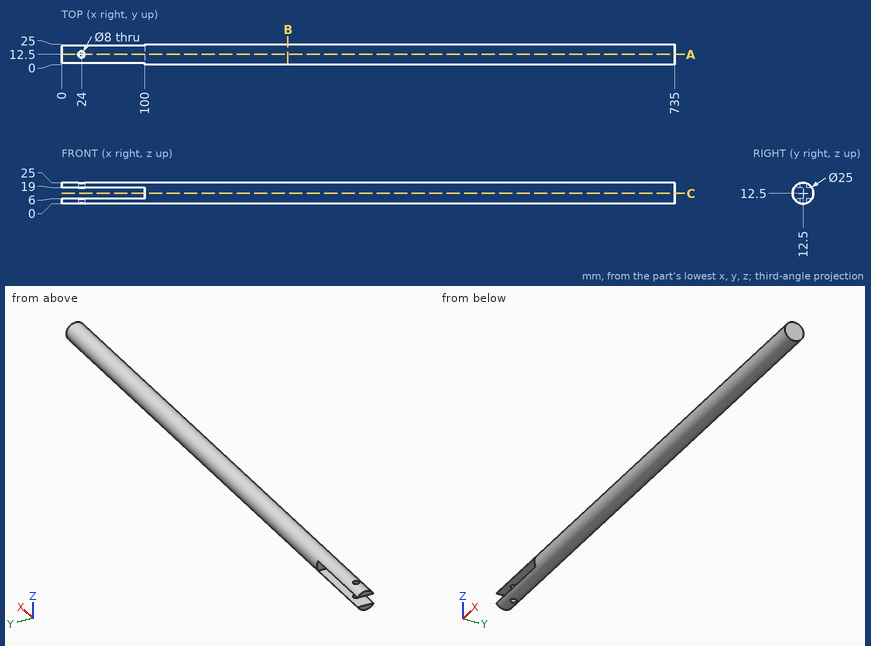
The drawing under review shows one solid part. Ordinate dimensions are in mm from its lowest x, y, z. Round coordinates to 2 decimals unless told otherwise and drop trailing zeros. Write each loop counter-clockwise with the first axis right and the second up, starting at its lowest first coordinate (ties: lowest second). Pieces come first, ordered by that corner, then holes. Notation, with made-up numbers: (43.25, 63) - (55.25, 63) arc R16 cw to (55.25, 83) - close; hole circle Ø10 at (-29, 53.5). An arc over 180 degrees is marked (long way). Put each result on its own line as item: value.
Q1. Insertion check: pin 1 Ø4 at (x, y) = (469.5, 11) entering from +Z; pin 2 Ø6 at (x, z) = (139, 19) entering from +Y; pin 3 Ø2 at (x, z) = (488.5, 16) entering from -Y; pin 4 Ø6.5 at (x, y) = (74, 8.5) entering from -Z. Each pin has a flat end and moves straight along its axis. Give the tip position at first contact, or say it passes through.
Solved:
pin 1: stops at z = 25
pin 2: stops at y = 24.5
pin 3: stops at y = 0.25
pin 4: stops at z = 0.02
Q2. We need section A-A (y = 12.5). Give the boundary of the cut face in (x, z).
Solved:
outline: (0, 0) - (20, 0) - (20, 6) - (0, 6) - close; (0, 19) - (20, 19) - (20, 25) - (0, 25) - close; (28, 0) - (735, 0) - (735, 25) - (28, 25) - (28, 19) - (100, 19) - (100, 6) - (28, 6) - close
Q3. Wall thickness on probe 1 along Y at (x, z) = (518, 6); probe 2 along X at (y, z) = (23.25, 9.5); probe 3 along Y at (x, z) = (24, 20.75): over which ranges is each line inside the solid? List them lowest first.
Solved:
probe 1: y = 1.82 to 23.18
probe 2: x = 100 to 735
probe 3: y = 3.11 to 8.5, 16.5 to 21.89
Q4. We need section C-C (z = 12.5). Give the boundary of the cut face in (x, y).
Solved:
outline: (100, 0) - (735, 0) - (735, 25) - (100, 25) - close
Q5. We need section B-B (x = 271.5). Give the boundary of the cut face in (y, z), and give its area (3 significant figures).
Solved:
outline: circle Ø25 at (12.5, 12.5)
area: 491 mm2
